Design review of the part built by this model. Coordinates are the model's own, in mm. Face numbers are marked on the shaded views. A direction names the side the tool comes from. Give positions to 0.01 mm unless a question says otherwise; leave off trailing zeros. Order: outer loops, then holes, each group sorted by start corner. A loop starts at its lowest first (then second) coordinate and runs counter-clockwise, first axis right, second up. Notation, with made-up numbers: M 34,73 L 40,73 A15 cw 40,78 Z; hole C 23,7 d5. An arc over 180 degrees is marked long. Answer as a JSON object with one key per item and string values.
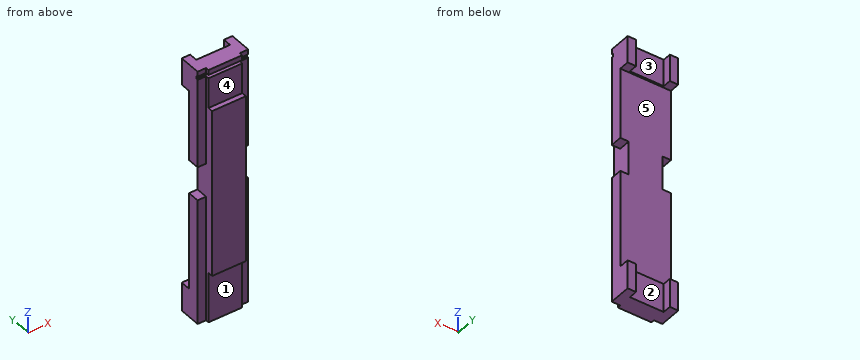
from build123d import *

# Parameters (mm, degrees)
SKETCH2_W           = 3
SKETCH2_H           = 15.3
BOSS_EXTRUDE1_DEPTH = 1.8
SKETCH3_W           = 12
SKETCH3_H           = 0.6
CUT_EXTRUDE1_DEPTH  = 4
SKETCH4_W           = 2.3
SKETCH4_H           = 0.3
SKETCH4_W_2         = 3
CUT_EXTRUDE2_DEPTH  = 4
SKETCH5_W           = 0.5
SKETCH5_H           = 2
CUT_EXTRUDE3_DEPTH  = 2.2
SKETCH8_W           = 2
SKETCH8_H           = 0.5
CUT_EXTRUDE5_DEPTH  = 16.3
SKETCH9_W           = 0.5
SKETCH9_H           = 0.5
CUT_EXTRUDE6_DEPTH  = 16.3
SKETCH10_W          = 0.2
SKETCH10_H          = 0.3
CUT_EXTRUDE7_DEPTH  = 4


with BuildPart() as part:
    # Sketch2 → Boss-Extrude1 (new body)
    with BuildSketch(Plane(origin=(0, 0, 0), x_dir=(1, 0, 0), z_dir=(0, 1, 0))):
        with Locations((0, 7.65)):
            Rectangle(SKETCH2_W, SKETCH2_H)
    extrude(amount=BOSS_EXTRUDE1_DEPTH)

    # Sketch3 → Cut-Extrude1 (cut, through all)
    with BuildSketch(Plane(origin=(1.5, 0, 0), x_dir=(0, 0, -1), z_dir=(1, 0, 0))):
        with Locations((7.6, 1.5)):
            Rectangle(SKETCH3_W, SKETCH3_H)
    extrude(amount=-CUT_EXTRUDE1_DEPTH, mode=Mode.SUBTRACT)

    # Sketch4 → Cut-Extrude2 (cut, through all)
    with BuildSketch(Plane(origin=(1.5, 0, 0), x_dir=(0, 0, -1), z_dir=(1, 0, 0))):
        with Locations((1.15, 0.15)):
            Rectangle(SKETCH4_W, SKETCH4_H)
        with Locations((13.8, 0.15)):
            Rectangle(SKETCH4_W_2, SKETCH4_H)
    extrude(amount=-CUT_EXTRUDE2_DEPTH, mode=Mode.SUBTRACT)

    # Sketch5 → Cut-Extrude3 (cut, through all)
    with BuildSketch(Plane(origin=(0, 1.2, 0), x_dir=(1, 0, 0), z_dir=(0, 1, 0))):
        with Locations((-1.25, 6.8)):
            Rectangle(SKETCH5_W, SKETCH5_H)
        with Locations((1.25, 6.8)):
            Rectangle(SKETCH5_W, SKETCH5_H)
    extrude(amount=-CUT_EXTRUDE3_DEPTH, mode=Mode.SUBTRACT)

    # Sketch8 → Cut-Extrude5 (cut, through all)
    with BuildSketch(Plane.XY):
        with Locations((0, 1.55)):
            Rectangle(SKETCH8_W, SKETCH8_H)
    extrude(amount=-CUT_EXTRUDE5_DEPTH, mode=Mode.SUBTRACT)

    # Sketch9 → Cut-Extrude6 (cut, through all)
    with BuildSketch(Plane.XY):
        with Locations((-1.25, 0.25)):
            Rectangle(SKETCH9_W, SKETCH9_H)
        with Locations((1.25, 0.25)):
            Rectangle(SKETCH9_W, SKETCH9_H)
    extrude(amount=-CUT_EXTRUDE6_DEPTH, mode=Mode.SUBTRACT)

    # Sketch10 → Cut-Extrude7 (cut, through all)
    with BuildSketch(Plane(origin=(1.5, 0, 0), x_dir=(0, 0, -1), z_dir=(1, 0, 0))):
        with Locations((0.4, 0.45)):
            Rectangle(SKETCH10_W, SKETCH10_H)
    extrude(amount=-CUT_EXTRUDE7_DEPTH, mode=Mode.SUBTRACT)


solid = part.part
(1) Insertion check: pin 1 (0.8 mm diameter, centred on x = -0.5, z = -1, fed in from +Y). The pin has a flat end and moves straight along its axis. Give the tip position at first contact, or say it passes through.
Checked values:
{"pin 1": "stops at y = 1.3"}
(2) Draft analysis for pull direction X (two halves, no side actions). For the marked faces 1 and 2, state which applies: +X half, -X half, draft (parallel to the pull), parting line (faces both ways), or undercut.
Checked values:
{"face 1": "draft", "face 2": "undercut"}
(3) We need section D-D (x = 0.25). Write out the cut boundary in (y, z).
Checked values:
{"outline": "M 0,-12.3 L 0.3,-12.3 L 0.3,-15.3 L 1.3,-15.3 L 1.3,-13.6 L 1.2,-13.6 L 1.2,-1.6 L 1.3,-1.6 L 1.3,0 L 0.3,0 L 0.3,-0.3 L 0.6,-0.3 L 0.6,-0.5 L 0.3,-0.5 L 0.3,-2.3 L 0,-2.3 Z"}
(4) Tool access review of the marked faces 3, 4 and 5: name each direction out of +Z, -Z, +X, -X, +Y, -Y from which nothing blocks a thin tool from reaching the whole face with its end or side.
Checked values:
{"face 3": "+Z, -Z, +Y", "face 4": "+Z, +X, -X, -Y", "face 5": "+X, -X, +Y"}
(5) We need section B-B (y = 0.9). Write out the cut boundary in (x, z).
Checked values:
{"outline": "M -1.5,-15.3 L 1.5,-15.3 L 1.5,-7.8 L 1,-7.8 L 1,-5.8 L 1.5,-5.8 L 1.5,0 L -1.5,0 L -1.5,-5.8 L -1,-5.8 L -1,-7.8 L -1.5,-7.8 Z"}
(6) To check wall thickness, follow L1, parallel to Z at x = 0.8, y = 0.55; L2, parallel to Z at x = -1.3, y = 0.9; L3, parallel to X at y = 0.5, z = -7.25. State the ranges of each line that lie inside material, in increasing order. Write a range as from..to.
Checked values:
{"L1": "z = -15.3..-0.5, -0.3..0", "L2": "z = -15.3..-7.8, -5.8..0", "L3": "x = -1..1"}
(7) We need section A-A (y = 1.55). Write out the cut boundary in (x, z).
Checked values:
{"outline": "M -1.5,-15.3 L -1,-15.3 L -1,-13.6 L -1.5,-13.6 Z; M -1.5,-1.6 L -1,-1.6 L -1,0 L -1.5,0 Z; M 1,-15.3 L 1.5,-15.3 L 1.5,-13.6 L 1,-13.6 Z; M 1,-1.6 L 1.5,-1.6 L 1.5,0 L 1,0 Z"}
(8) We need section C-C (z = -4). Write out the cut boundary in (x, y).
Checked values:
{"outline": "M -1.5,0.5 L -1,0.5 L -1,0 L 1,0 L 1,0.5 L 1.5,0.5 L 1.5,1.2 L -1.5,1.2 Z"}
